from build123d import *

# Parameters (mm, degrees)
F0_R     = 2.38125
F1_DEPTH = 6.35
F3_DEPTH = 25.4


with BuildPart() as f1:
    # F0 (on Right) → F1 (new body)
    with BuildSketch(Plane.YZ):
        with BuildLine():
            Line((460.375, 9.525), (0, 9.525))
            ThreePointArc((0, 9.525), (-9.525, 0), (0, -9.525))
            Line((0, -9.525), (460.375, -9.525))
            ThreePointArc((460.375, -9.525), (469.9, 0), (460.375, 9.525))
        make_face()
        Circle(F0_R, mode=Mode.SUBTRACT)
        with Locations((323.85, 0)):
            Circle(F0_R, mode=Mode.SUBTRACT)
        with Locations((460.375, 0)):
            Circle(F0_R, mode=Mode.SUBTRACT)
    extrude(amount=F1_DEPTH)

    # F2 (on face) → F3 (cut)
    with BuildSketch(Plane.XY.offset(9.525)):
        Polygon((3.175, 298.47035), (6.35, 50.8), (6.35, 469.9), (3.175, 469.9), align=None)
        Polygon((3.175, 50.77965), (0, 298.45), (0, -9.525), (3.175, -9.525), align=None)
    extrude(amount=-F3_DEPTH, mode=Mode.SUBTRACT)


solid = f1.part
Input: part model. Units: mm. Frame: model coordinates. A direction names the side the tool comes from. Give positions to 0.01 mm unless a question says otherwise; leave off trailing zeros. Write each loop counter-clockwise with the first axis right and the second up, starting at its lowest first coordinate (ties: lowest second). Pieces come first, ordered by that corner, then holes. Notation, with made-up numbers: M -23.75,36 L 19.25,36 A32 cw 19.25,70 Z; hole C 2,77.5 d5. An arc over 180 degrees is marked long. Use one line per item in the form item = value.
1. Cut plane A-A on z = 6.25. Return loops of the section in (x, y) (3 decimals), and give its area (3 significant figures).
Outcome:
outline = M 0,298.45 L 3.175,50.78 L 3.175,-7.188 L 6.35,-7.188 L 6.35,50.8 L 3.175,298.47 L 3.175,467.563 L 0,467.563 Z
area = 1,510 mm²
2. Reachability of faces 1 (the face through (1.565, 469.898, -0.209)), 2 (the face through (3.175, 20, 0)), 3 (the face through (3.175, 385, 0)) from +Z, -Z, +X, -X, +Y, -Y: full face, straight path, thin tool, end or side. Return the list, or none.
Outcome:
face_1 = +X, -X, +Y
face_2 = +Z, -Z, -X, -Y
face_3 = +Z, -Z, +X, +Y
3. Ray query, L1, parallel to X at y = 431.5, z = -5.75 (3 decimals); L2, parallel to Z at x = 1.45, y = 323.85 (3 decimals); L3, parallel to X at y = 25, z = -5.25 (3 decimals). Return the intervals inside material, ascending.
Outcome:
L1 = 0 to 3.175
L2 = -9.525 to -2.381, 2.381 to 9.525
L3 = 3.175 to 6.35
4. Cut plane B-B on y = 355.5. Return loops of the section in (x, z) (3 decimals).
Outcome:
outline = M 0,-9.525 L 3.175,-9.525 L 3.175,9.525 L 0,9.525 Z
5. Cut plane C-C on y = 73.5. Return loops of the section in (x, z) (3 decimals).
Outcome:
outline = M 2.884,-9.525 L 6.059,-9.525 L 6.059,9.525 L 2.884,9.525 Z
6. First-contact query: P1, Ø8, axis at y = 381.5, z = 6.5, coming from the -X side; P2, Ø10, axis at y = 131.5, z = -3, coming from the -X side; P3, Ø1.5, axis at y = 201, z = 5.5, coming from the -X side. Flat tips, straight axial feed; report the tip coordinate or a pass-through.
Outcome:
P1 = 0
P2 = 2.08
P3 = 1.24
